Could you check a few things on this model? Use its own coordinates, in mm. Coordinates: 2 decimals unless noted, no trailing zeros. Loops run counter-clockwise (first coordinate to the right, second up) from the corner with the lowest first, then second, coordinate; pieces in that order, holes last. Notation, with made-up numbers: M -6,-17 L 20,-17 A36 cw 20,20 Z; hole C 58,71.25 d5. An arc over 180 degrees is marked long. Use one line per item in the form item = value. Start each with the question number.
```python
from build123d import *

# Parameters (mm, degrees)
SKETCH_1_W      = 6.1
SKETCH_1_H      = 6.1
SKETCH_1_R      = 9.55
SKETCH_1_R_2    = 2.55
EXTRUDE_2_DEPTH = 2
FILLET_1_R      = 45
FILLET_2_R      = 10


with BuildPart() as part:
    # 草图1 → 凸台-拉伸2 (new body)
    with BuildSketch(Plane.XY):
        with BuildLine():
            Line((-10.195923298, 166.045688989), (-10.195923298, 93.338899377))
            Line((-10.195923298, 93.338899377), (-10.195923298, -3.112918115))
            Line((-10.195923298, -3.112918115), (6.754076702, -25.161100623))
            ThreePointArc((6.754076702, -25.161100623), (31.304076702, -49.711100623), (55.854076702, -25.161100623))
            Line((55.854076702, -25.161100623), (61.387071712, 1.202006387))
            Line((61.387071712, 1.202006387), (61.387071712, 34.710258927))
            Line((61.387071712, 34.710258927), (52.804076702, 50.954174352))
            Line((52.804076702, 50.954174352), (52.804076702, 93.338899377))
            Line((52.804076702, 93.338899377), (52.804076702, 205.407441872))
            Line((52.804076702, 205.407441872), (0, 234.171513377))
            ThreePointArc((0, 234.171513377), (-34.1851727, 217.056026281), (-10.195923298, 187.288899377))
            Line((-10.195923298, 187.288899377), (-10.195923298, 166.045688989))
        make_face()
        with Locations((10.304076702, 14.560258927)):
            Rectangle(SKETCH_1_W, SKETCH_1_H, mode=Mode.SUBTRACT)
        with Locations((10.304076702, 31.660258927)):
            Rectangle(SKETCH_1_W, SKETCH_1_H, mode=Mode.SUBTRACT)
        with Locations((31.304076702, -25.161100623)):
            Circle(SKETCH_1_R, mode=Mode.SUBTRACT)
        with Locations((26.304076702, 19.560258927)):
            Circle(SKETCH_1_R_2, mode=Mode.SUBTRACT)
        with Locations((36.304076702, 19.560258927)):
            Circle(SKETCH_1_R_2, mode=Mode.SUBTRACT)
        with Locations((52.304076702, 14.560258927)):
            Rectangle(SKETCH_1_W, SKETCH_1_H, mode=Mode.SUBTRACT)
        with Locations((52.304076702, 31.660258927)):
            Rectangle(SKETCH_1_W, SKETCH_1_H, mode=Mode.SUBTRACT)
        Polygon((7.355428358, 168.902414276), (3.042076993, 164.589062911), (-1.271274372, 168.902414276), (3.042076993, 173.215765641), align=None, mode=Mode.SUBTRACT)
        with Locations((-10.195923298, 211.838899377)):
            Circle(SKETCH_1_R, mode=Mode.SUBTRACT)
        Polygon((40.518736396, 42.143243143), (7.254076702, 42.143243143), (7.254076702, 134.668841545), (40.518736396, 162.856651297), align=None, mode=Mode.SUBTRACT)
        Polygon((19.446954316, 156.810888318), (15.133602951, 152.497536952), (10.820251586, 156.810888318), (15.133602951, 161.124239683), align=None, mode=Mode.SUBTRACT)
        with Locations((17.891319398, 176.680588869)):
            Circle(SKETCH_1_R_2, mode=Mode.SUBTRACT)
        with Locations((24.96238721, 183.751656681)):
            Circle(SKETCH_1_R_2, mode=Mode.SUBTRACT)
        Polygon((32.740561803, 202.914250451), (37.053913168, 198.600899086), (32.740561803, 194.28754772), (28.427210437, 198.600899086), align=None, mode=Mode.SUBTRACT)
        Polygon((49.145439126, 186.509373127), (44.832087761, 182.196021762), (40.518736396, 186.509373127), (44.832087761, 190.822724493), align=None, mode=Mode.SUBTRACT)
    extrude(amount=EXTRUDE_2_DEPTH)

    # 圆角1
    fillet_1_edges = [part.edges().sort_by_distance(p)[0] for p in [
        (52.804076702, 205.407441872, 1),
        (52.804076702, 50.954174352, 1),
        (-10.195923298, -3.112918115, 1),
    ]]
    fillet(fillet_1_edges, radius=FILLET_1_R)

    # 圆角2
    fillet_2_edges = [part.edges().sort_by_distance(p)[0] for p in [
        (40.518736396, 162.856651297, 1),
        (7.254076702, 134.668841545, 1),
        (7.254076702, 42.143243143, 1),
        (40.518736396, 42.143243143, 1),
        (-10.195923298, 187.288899377, 1),
    ]]
    fillet(fillet_2_edges, radius=FILLET_2_R)


solid = part.part
```
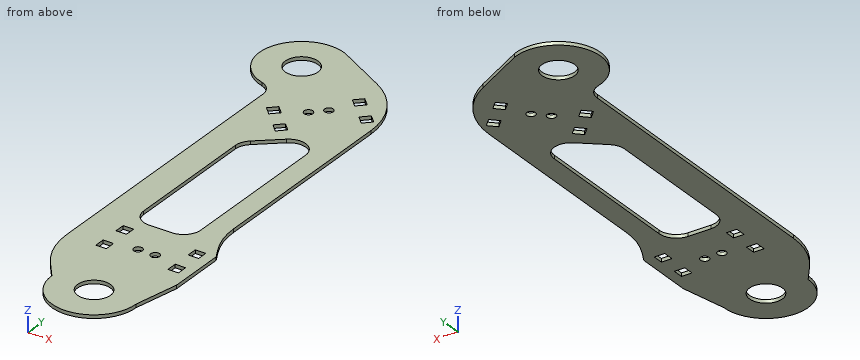
Item 1: Please list where these lines run through material, in increasing order: line 1 along X through (y, z) = (14.5, 0.55); line 2 along X through (y, z) = (18, 1.95); line 3 along X through (y, z) = (75.5, 0.4).
Item 2: I want a section at A-A (y = 81.5). Write out the boundary of the cut face in (x, z).
Item 3: I want a section at B-B (z = 1.5). Count the separate pieces of the cut face and the enclosed holes in it, plus the area to 3 significant figures.
Item 4: I'm going to push flat-ended pins straight in: P1, Ø17, axis at x = 31.3, y = -25.16, coming from the -Z side; P2, Ø1, axis at x = 34.5, z = 1, coming from the -Y side; P3, Ø0.6, axis at y = 14, z = 1, coming from the -X side; P4, Ø0.6, axis at x = 11.5, z = 1, coming from the -Y side. Where does each tip first touch, or does it pass through?
Worked answers:
q1.line_1 = -10.2 to 7.25, 13.35 to 49.25, 55.35 to 61.39
q1.line_2 = -10.2 to 24.29, 28.32 to 34.29, 38.32 to 61.39
q1.line_3 = -10.2 to 7.25, 40.52 to 52.8
q2.outline = M -10.2,0 L 7.25,0 L 7.25,2 L -10.2,2 Z; M 40.52,0 L 52.8,0 L 52.8,2 L 40.52,2 Z
q3.separate_pieces = 1
q3.enclosed_holes = 15
q3.area = 13,300 mm²
q4.P1 = through
q4.P2 = -49.56
q4.P3 = -10.2
q4.P4 = -40.07
